Read the model definition and answer for the solid it produces. Units are mm, in the model's axes. Coordinates: 2 decimals unless noted, no trailing zeros. Write each loop counter-clockwise with the first axis right and the second up, starting at its lowest first coordinate (ties: lowest second). Pieces come first, ordered by that corner, then holes. Notation, with made-up numbers: (-13.75, 4.25) - (11.25, 4.25) arc R19 cw to (11.25, 29.25) - close; hole circle Ø8 at (-2, -16.75). An arc over 180 degrees is marked (long way). Return JSON: item names as keys, results as strings.
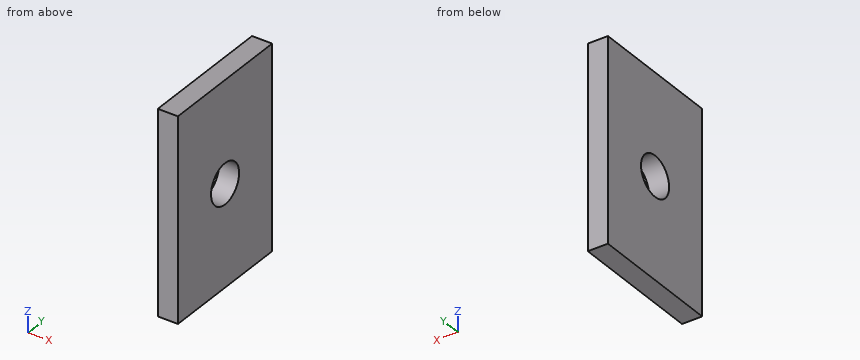
```python
from build123d import *

# Parameters (mm, degrees)
F0_W     = 73.6056677997
F0_H     = 50.1926615834
F0_R     = 5
F1_DEPTH = 5
F3_DEPTH = 20
F4_DEPTH = 20


with BuildPart() as f1:
    # F0 (on Right) → F1 (new body)
    with BuildSketch(Plane.YZ):
        with Locations((-64.2384514213, 25.0963307917)):
            Rectangle(F0_W, F0_H)
        with Locations((-64.2384514213, 25.0963307917)):
            Circle(F0_R, mode=Mode.SUBTRACT)
    extrude(amount=F1_DEPTH)

    # F3 (cut): a face of the model
    f3_faces = [f1.faces().sort_by_distance(p)[0] for p in [
        (2.5, -101.0412853211, 25.0963307917),
    ]]
    extrude(f3_faces, amount=-F3_DEPTH, mode=Mode.SUBTRACT)

    # F4 (cut): a face of the model
    f4_faces = [f1.faces().sort_by_distance(p)[0] for p in [
        (2.5, -27.4356175214, 25.0963307917),
    ]]
    extrude(f4_faces, amount=-F4_DEPTH, mode=Mode.SUBTRACT)


solid = f1.part
```
(1) A cutting plane is placed at B-B (y = -62). Determine the outline of the cut face in (x, z).
Answer:
{"outline": "(0, 0) - (5, 0) - (5, 20.63) - (0, 20.63) - close; (0, 29.57) - (5, 29.57) - (5, 50.19) - (0, 50.19) - close"}
(2) A cutting plane is placed at A-A (z = 24.5). Determine the outline of the cut face in (x, y).
Answer:
{"outline": "(0, -81.04) - (5, -81.04) - (5, -69.2) - (0, -69.2) - close; (0, -59.27) - (5, -59.27) - (5, -47.44) - (0, -47.44) - close"}
(3) A cutting plane is placed at C-C (x = 2.75). Determine the outline of the cut face in (y, z), and give its area (3 significant figures).
Answer:
{"outline": "(-81.04, 0) - (-47.44, 0) - (-47.44, 50.19) - (-81.04, 50.19) - close; hole circle Ø10 at (-64.24, 25.1)", "area": "1,610 mm²"}
(4) Flat-ended cylindrical pins translate along their axes: P1, Ø12, axis at y = -57, z = 14, coming from the -X side; P2, Ø1.5, axis at y = -63, z = 21.5, coming from the -X side. Find the tip coordinate at first contact, or state that the pin passes through.
Answer:
{"P1": "x = 0", "P2": "through"}
(5) Straight lines are drawn through the part: line 1 (Z direction, x = 1.75, y = -61.5); line 2 (Y direction, x = 2.6, z = 28.5); line 3 (Z direction, x = 1.8, y = -66.5). For each, find the intervals that lie inside material, in ascending order. Write a range as from..to.
Answer:
{"line 1": "0..20.91, 29.28..50.19", "line 2": "-81.04..-67.9, -60.58..-47.44", "line 3": "0..20.64, 29.56..50.19"}
